Verification items for the finished model (mm, model axes). Face numbers are marked on the shaded views. A direction names the side the tool comes from. Coordinates: 2 decimals unless noted, no trailing zeros. Loops run counter-clockwise (first coordinate to the right, second up) from the corner with the lowest first, then second, coordinate; pieces in that order, holes last. Notation, with made-up numbers: (-1.75, 29.25) - (23.25, 29.25) arc R5 cw to (23.25, 33.25) - close; hole circle Ø6 at (80, -25.75). An arc over 180 degrees is marked (long way). Answer as CSV lines item,"result". Start each with the question number.
1. Cross-section at A-A (x = 30). Enter the section's corners in (y, z).
2. Cross-section at D-D (y = 22). State how many separate pieces and enclosed holes the cut face has, plus the area to 3 significant figures.
3. Set-up check for the marked faces 1 and 2: record each of +Z, -Z, +X, -X, +Y, -Y from which the full face is reachable in a straight line by a thin tool's end or side.
4. Gauge pin test, flat ends, axial feed: P1, Ø6, axis at y = 42.5, z = -63, coming from the -X side; P2, Ø6, axis at y = 17, z = 52, coming from the +X side; P3, Ø0.9, axis at x = 1.5, z = 55, coming from the +Y side; P4, Ø1.5, axis at x = 19.5, z = -50, coming from the +Y side. Record the tip position at first contact, or that the pin passes through.
5. Material ranges on line 1 (Y direction, x = 1.35, z = 15.5); line 2 (Y direction, x = 1, z = 15); line 3 (Y direction, x = 2.15, z = -55), recorded low to high. Write a range as [from, to].
6. Cross-section at C-C (z = -55). Enter the section's corners in (x, y).
7. Cross-section at B-B (y = 6.5). Enter the section's corners in (x, z), plus the area to 3 significant figures.
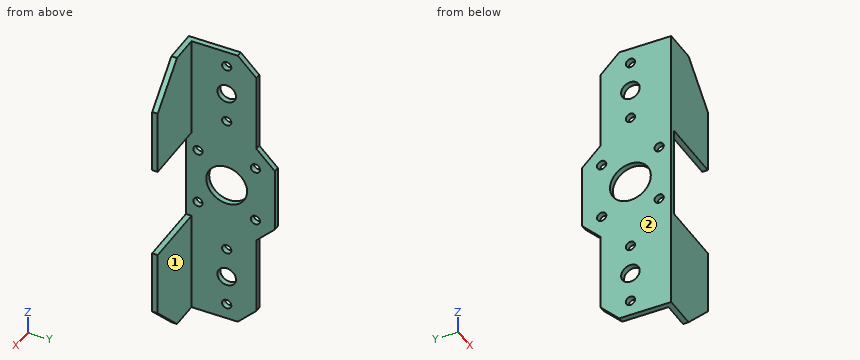
```python
from build123d import *

# Parameters (mm, degrees)
SALIENTE_EXTRUIR1_DEPTH      = 80
SALIENTE_EXTRUIR1_DEPTH_BACK = 80
CROQUIS2_W                   = 35
CROQUIS2_H                   = 50
CORTAR_EXTRUIR1_DEPTH        = 3
CHAFL_N1_SIZE                = 20
CROQUIS3_R                   = 5
CROQUIS3_R_2                 = 2.5
CORTAR_EXTRUIR2_DEPTH        = 3
CROQUIS4_W                   = 55
CROQUIS4_H                   = 10
SALIENTE_EXTRUIR2_DEPTH      = 3
CROQUIS5_R                   = 2.5
CROQUIS5_R_2                 = 11
CORTAR_EXTRUIR3_DEPTH        = 3
CHAFL_N2_SIZE                = 10


with BuildPart() as part:
    # Croquis1 → Saliente-Extruir1 (new, two sides: drawn at the far end of the back side and taken through both)
    with BuildSketch(Plane.XY.offset(-SALIENTE_EXTRUIR1_DEPTH_BACK)):
        Polygon((0, 0), (0, 38), (3, 38), (3, 3), (38, 3), (38, 0), align=None)
    extrude(amount=SALIENTE_EXTRUIR1_DEPTH + SALIENTE_EXTRUIR1_DEPTH_BACK)

    # Croquis2 → Cortar-Extruir1 (cut)
    with BuildSketch(Plane(origin=(0, 3, 0), x_dir=(1, 0, 0), z_dir=(0, 1, 0))):
        with Locations((20.5, 0)):
            Rectangle(CROQUIS2_W, CROQUIS2_H)
    extrude(amount=-CORTAR_EXTRUIR1_DEPTH, mode=Mode.SUBTRACT)

    # Chaflán1
    chafl_n1_edges = [part.edges().sort_by_distance(p)[0] for p in [
        (38, 1.5, 80),
        (38, 1.5, -80),
    ]]
    chamfer(chafl_n1_edges, length=CHAFL_N1_SIZE)

    # Croquis3 → Cortar-Extruir2 (cut)
    with BuildSketch(Plane(origin=(3, 0, 0), x_dir=(0, 0, -1), z_dir=(1, 0, 0))):
        with Locations((-55, 22)):
            Circle(CROQUIS3_R)
        with Locations((-71.5, 22)):
            Circle(CROQUIS3_R_2)
        with Locations((-38.5, 22)):
            Circle(CROQUIS3_R_2)
        with Locations(Location((38.5, 22, 0), (0, 0, 180))):
            Circle(CROQUIS3_R_2)
        with Locations(Location((55, 22, 0), (0, 0, 180))):
            Circle(CROQUIS3_R)
        with Locations(Location((71.5, 22, 0), (0, 0, 180))):
            Circle(CROQUIS3_R_2)
    extrude(amount=-CORTAR_EXTRUIR2_DEPTH, mode=Mode.SUBTRACT)

    # Croquis4 → Saliente-Extruir2 (add)
    with BuildSketch(Plane.ZY):
        with Locations((0, 43)):
            Rectangle(CROQUIS4_W, CROQUIS4_H)
    extrude(amount=-SALIENTE_EXTRUIR2_DEPTH)

    # Croquis5 → Cortar-Extruir3 (cut)
    with BuildSketch(Plane.ZY):
        with Locations((-15.5, 37.5)):
            Circle(CROQUIS5_R)
        with Locations((15.5, 37.5)):
            Circle(CROQUIS5_R)
        with Locations((15.5, 6.5)):
            Circle(CROQUIS5_R)
        with Locations((-15.5, 6.5)):
            Circle(CROQUIS5_R)
        with Locations((0, 22)):
            Circle(CROQUIS5_R_2)
    extrude(amount=-CORTAR_EXTRUIR3_DEPTH, mode=Mode.SUBTRACT)

    # Chaflán2
    chafl_n2_edges = [part.edges().sort_by_distance(p)[0] for p in [
        (1.5, 38, 80),
        (1.5, 38, -80),
        (1.5, 48, -27.5),
        (1.5, 48, 27.5),
    ]]
    chamfer(chafl_n2_edges, length=CHAFL_N2_SIZE - 0.0001)  # a hair under: the kernel refuses the full size


solid = part.part
```
Values follow:
1,outline,"(0, -68) - (3, -68) - (3, -25) - (0, -25) - close; (0, 25) - (3, 25) - (3, 68) - (0, 68) - close"
2,separate pieces,"8"
2,enclosed holes,"0"
2,area,"294 mm²"
3,face 1,"+Z, -Z, +X, +Y"
3,face 2,"+Z, -Z, -X, +Y, -Y"
4,P1,"passes through"
4,P2,"stops at x = 3"
4,P3,"stops at y = 38"
4,P4,"stops at y = 3"
5,line 1,"y = [0, 4], [9, 35], [40, 48]"
5,line 2,"y = [0, 4.05], [8.95, 35.05], [39.95, 48]"
5,line 3,"y = [0, 17], [27, 38]"
6,outline,"(0, 0) - (38, 0) - (38, 3) - (3, 3) - (3, 17) - (0, 17) - close; (0, 27) - (3, 27) - (3, 38) - (0, 38) - close"
7,outline,"(0, -80) - (3, -80) - (3, -18) - (0, -18) - close; (0, -13) - (3, -13) - (3, 13) - (0, 13) - close; (0, 18) - (3, 18) - (3, 80) - (0, 80) - close"
7,area,"450 mm²"
